Here's how the part is built. I have some questions about the finished solid (model axes, mm). Face numbers are marked on the shaded views. A direction names the side the tool comes from. Coordinates: 2 decimals unless noted, no trailing zeros. Write each loop counter-clockwise with the first axis right and the second up, starting at its lowest first coordinate (ties: lowest second). Pieces come first, ordered by that corner, then holes. Notation, with made-up numbers: (-4, 55.5) -> (35, 55.5) arc R36 ccw to (35, 92.5) -> close; hole circle Ø7 at (-25.5, -7). An arc over 180 degrees is marked (long way). Put each result on its own line as item: value. Start each with the question number.
Item 1: I need wall thicknesses on line 1 (X direction, y = 11.35, z = 8.85); line 2 (X direction, y = 7, z = 0); line 3 (X direction, y = 3.5, z = 9.25). Which ranges of each line are inside material? Lowest first, please. Write a range as [from, to].
Item 2: I want a section at A-A, the plane y = 7. List the corners of the cut face in (x, z) for me.
Item 3: I want a section at B-B, the plane z = -8.85. List the corners of the cut face in (x, y) for me, then the cut area to 3 significant figures.
Item 4: I want a section at C-C, the plane y = -6. List the corners of the cut face in (x, z) for me, then the cut area to 3 significant figures.
Item 5: I want a section at D-D, the plane x = 27. List the corners of the cut face in (y, z) for me, then the cut area to 3 significant figures.
Item 6: On a 3-axis mill with a long thin cutter (end or side, diameter ignored), from which of +Z, -Z, +X, -X, +Y, -Y can I reach the whole of each face in a straight line? I mean the marked faces 4, 5, 6 and 7. Say none if no direction works.
Item 7: If we mould it in two halves opening along X, with no side actions, what happens to the marked faces 1, 2 and 3? For each: released by +X, released by -X, zero draft, split by the parting line, or undercut.
Item 8: For pin 1 (1.1 mm diameter, centred on x = 30, y = -9.5, fed in from -Z); pin 2 (3 mm diameter, centred on x = -21.35, z = -8.85, fed in from -Y); pin 3 (13 mm diameter, centred on y = 7.5, z = -2.5, fed in from -X), each with a flat end and sliding along its axis, tell me the tip position at first contact or that it passes through.
from build123d import *

# Parameters (mm, degrees)
SKETCH1_W           = 52
SKETCH1_H           = 24
SKETCH1_R           = 8.25
BOSS_EXTRUDE1_DEPTH = 12
SKETCH2_R           = 1
CUT_EXTRUDE1_DEPTH  = 32.048349393
SKETCH3_R           = 1.75
CUT_EXTRUDE2_DEPTH  = 1
CUT_EXTRUDE3_DEPTH  = 5
FILLET3_R           = 0.5
CHAMFER1_SIZE       = 2.5
SKETCH5_W           = 14
SKETCH5_H           = 8
CUT_EXTRUDE4_DEPTH  = 5
FILLET4_R           = 0.5
BOSS_EXTRUDE2_DEPTH = 7
BOSS_EXTRUDE3_START = -52
BOSS_EXTRUDE3_DEPTH = 7
CHAMFER2_SIZE       = 2.5


with BuildPart() as part:
    # Sketch1 → Boss-Extrude1 (new body)
    with BuildSketch(Plane(origin=(0, 0, 0), x_dir=(1, 0, 0), z_dir=(0, 1, 0))):
        Rectangle(SKETCH1_W, SKETCH1_H)
        with Locations(Location((12.75, 0, 0), (0, 0, 270))):
            Circle(SKETCH1_R, mode=Mode.SUBTRACT)
        with Locations(Location((-12.75, 0, 0), (0, 0, 270))):
            Circle(SKETCH1_R, mode=Mode.SUBTRACT)
    extrude(amount=BOSS_EXTRUDE1_DEPTH)

    # Sketch2 → Cut-Extrude1 (cut, through all)
    with BuildSketch(Plane(origin=(0, 12, 0), x_dir=(1, 0, 0), z_dir=(0, 1, 0))):
        with Locations(Location((-21.35, 8.85, 0), (0, 0, 270))):
            Circle(SKETCH2_R)
        with Locations(Location((21.35, 8.85, 0), (0, 0, 270))):
            Circle(SKETCH2_R)
        with Locations(Location((21.35, -8.85, 0), (0, 0, 270))):
            Circle(SKETCH2_R)
        with Locations(Location((-21.35, -8.85, 0), (0, 0, 270))):
            Circle(SKETCH2_R)
    extrude(amount=-CUT_EXTRUDE1_DEPTH, mode=Mode.SUBTRACT)

    # Sketch3 → Cut-Extrude2 (cut)
    with BuildSketch(Plane(origin=(0, 12, 0), x_dir=(1, 0, 0), z_dir=(0, 1, 0))):
        with Locations(Location((-21.35, 8.85, 0), (0, 0, 270))):
            Circle(SKETCH3_R)
        with Locations(Location((21.35, 8.85, 0), (0, 0, 270))):
            Circle(SKETCH3_R)
        with Locations(Location((21.35, -8.85, 0), (0, 0, 270))):
            Circle(SKETCH3_R)
        with Locations(Location((-21.35, -8.85, 0), (0, 0, 270))):
            Circle(SKETCH3_R)
    extrude(amount=-CUT_EXTRUDE2_DEPTH, mode=Mode.SUBTRACT)

    # Sketch4 → Cut-Extrude3 (cut)
    with BuildSketch(Plane.XZ):
        Polygon((-6, -5), (-6, -12), (6, -12), (6, -5), (0, -5), align=None)
    extrude(amount=-CUT_EXTRUDE3_DEPTH, mode=Mode.SUBTRACT)

    # Fillet3
    fillet3_edges = [part.edges().sort_by_distance(p)[0] for p in [
        (-6, 2.5, -5),
        (6, 5, -8.5),
        (6, 2.5, -5),
        (-6, 5, -8.5),
        (0, 5, -5),
    ]]
    fillet(fillet3_edges, radius=FILLET3_R)

    # Chamfer1
    chamfer1_edges = [part.edges().sort_by_distance(p)[0] for p in [
        (26, 6, 12),
        (-26, 6, 12),
        (-26, 6, -12),
        (26, 6, -12),
    ]]
    chamfer(chamfer1_edges, length=CHAMFER1_SIZE)

    # Sketch5 → Cut-Extrude4 (cut)
    with BuildSketch(Plane.XZ):
        with Locations((0, 12)):
            Rectangle(SKETCH5_W, SKETCH5_H)
    extrude(amount=-CUT_EXTRUDE4_DEPTH, mode=Mode.SUBTRACT)

    # Fillet4
    fillet4_edges = [part.edges().sort_by_distance(p)[0] for p in [
        (-7, 2.5, 8),
        (7, 5, 10),
        (0, 5, 8),
        (-7, 5, 10),
        (7, 2.5, 8),
    ]]
    fillet(fillet4_edges, radius=FILLET4_R)

    # Sketch6 → Boss-Extrude2 (add)
    with BuildSketch(Plane(origin=(26, 0, 0), x_dir=(0, 0, -1), z_dir=(1, 0, 0))):
        Polygon((-5.5, 0), (-5.5, 12), (-9.5, 12), (-9.5, -10.909520595), (-2, -10.909520595), (-2, -7.309520595), (-5.5, -7.309520595), align=None)
    extrude(amount=BOSS_EXTRUDE2_DEPTH)

    # Sketch6<2> → Boss-Extrude3 (add)
    with BuildSketch(Plane(origin=(26, 0, 0), x_dir=(0, 0, -1), z_dir=(1, 0, 0)).offset(BOSS_EXTRUDE3_START)):
        Polygon((-5.5, 0), (-5.5, 12), (-9.5, 12), (-9.5, -10.909520595), (-2, -10.909520595), (-2, -7.309520595), (-5.5, -7.309520595), align=None)
    extrude(amount=-BOSS_EXTRUDE3_DEPTH)

    # Chamfer2
    chamfer2_edges = [part.edges().sort_by_distance(p)[0] for p in [
        (29.5, -10.909520595, 9.5),
        (-29.5, -10.909520595, 9.5),
    ]]
    chamfer(chamfer2_edges, length=CHAMFER2_SIZE)


solid = part.part
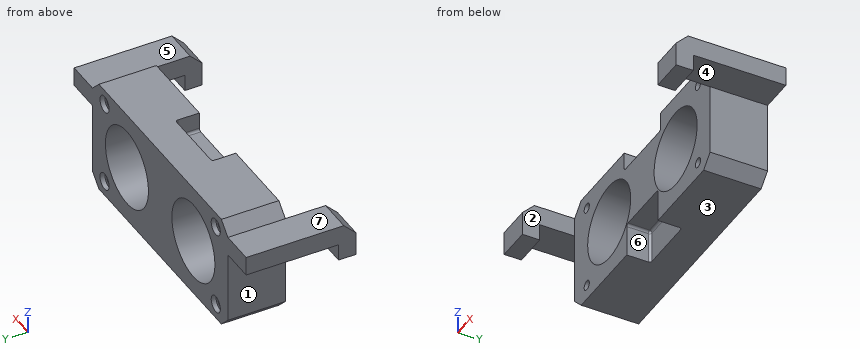
Calculated:
1. line 1: x = [-33, -23.1], [-19.6, 19.6], [23.1, 33]
1. line 2: x = [-26, -21], [-4.5, 4.5], [21, 26]
1. line 3: x = [-33, -22.27], [-20.43, -7], [7, 20.43], [22.27, 33]
2. outline: (-33, 5.5) -> (-26, 5.5) -> (-26, -9.5) -> (-23.5, -12) -> (23.5, -12) -> (26, -9.5) -> (26, 5.5) -> (33, 5.5) -> (33, 9.5) -> (26, 9.5) -> (23.5, 12) -> (-23.5, 12) -> (-26, 9.5) -> (-33, 9.5) -> close; hole circle Ø2 at (-21.35, -8.85); hole circle Ø2 at (-21.35, 8.85); hole circle Ø16.5 at (-12.75, 0); hole circle Ø16.5 at (12.75, 0); hole circle Ø2 at (21.35, -8.85); hole circle Ø2 at (21.35, 8.85)
3. outline: (-26, 0) -> (-22.35, 0) -> (-22.35, 11) -> (-23.1, 11) -> (-23.1, 12) -> (-26, 12) -> close; (-20.35, 0) -> (-6, 0) -> (-6, 4.5) arc R0.5 cw to (-5.5, 5) -> (5.5, 5) arc R0.5 cw to (6, 4.5) -> (6, 0) -> (20.35, 0) -> (20.35, 11) -> (19.6, 11) -> (19.6, 12) -> (-19.6, 12) -> (-19.6, 11) -> (-20.35, 11) -> close; (22.35, 0) -> (26, 0) -> (26, 12) -> (23.1, 12) -> (23.1, 11) -> (22.35, 11) -> close
3. area: 513 mm2
4. outline: (-33, 5.5) -> (-26, 5.5) -> (-26, 9.5) -> (-33, 9.5) -> close; (26, 5.5) -> (33, 5.5) -> (33, 9.5) -> (26, 9.5) -> close
4. area: 56.0 mm2
5. outline: (-10.91, 2) -> (-7.31, 2) -> (-7.31, 5.5) -> (12, 5.5) -> (12, 9.5) -> (-8.41, 9.5) -> (-10.91, 7) -> close
5. area: 101 mm2
6. face 4: -Z, +X, +Y
6. face 5: +Z, +X, +Y, -Y
6. face 6: -Z, -Y
6. face 7: +Z, -X, +Y, -Y
7. face 1: released by -X
7. face 2: undercut
7. face 3: zero draft
8. pin 1: stops at z = 2
8. pin 2: stops at y = 0
8. pin 3: stops at x = -26
